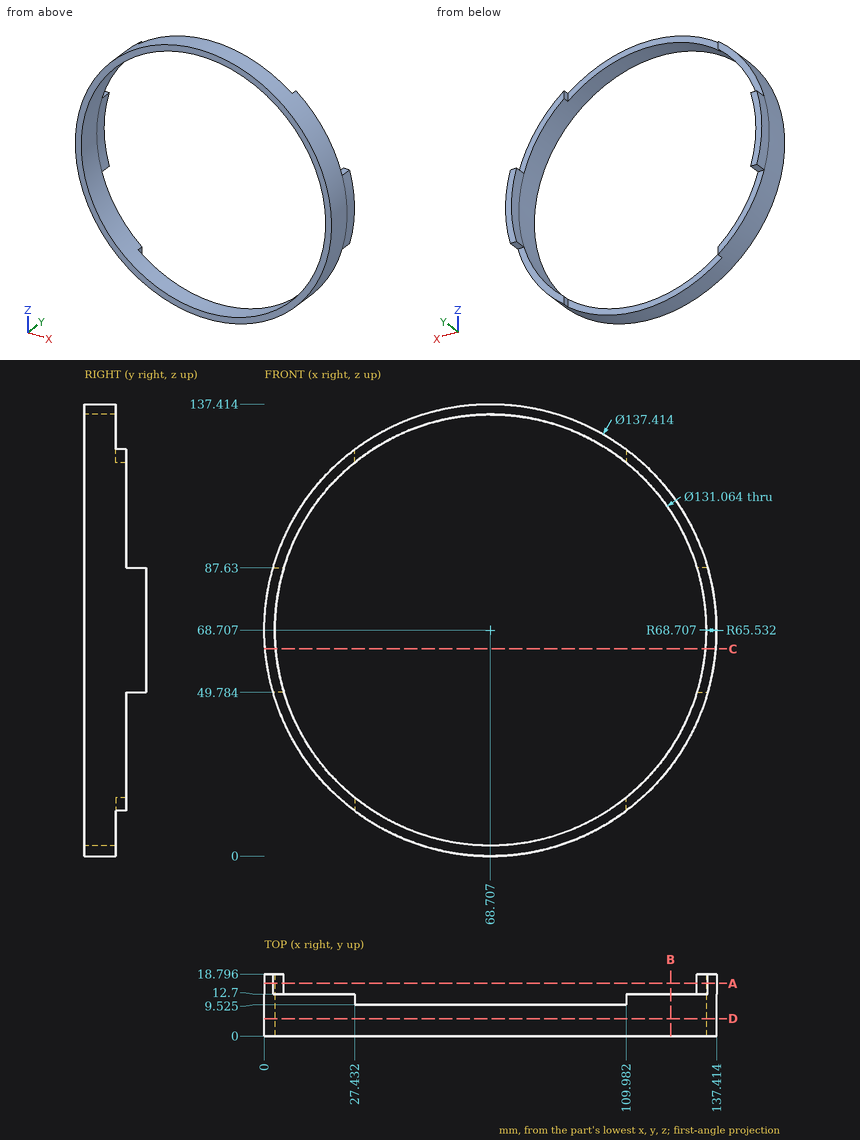
Can you work these out from the drawing? Everything is in mm from the part's minimum corner. Give positions to 0.01 mm unless a question says otherwise; leave off trailing zeros. Order: outer loops, then holes, each group sorted by start corner. A loop starts at its lowest first (then second) coordinate and runs counter-clockwise, first axis right, second up.
Item 1: If we section it at C-C, the plane z = 63: Write out the boundary of the cut face in (x, y), plus the area to 3 significant figures.
Item 2: If we section it at B-B, the plane x = 123.5: Write out the boundary of the cut face in (y, z), plus the area to 3 significant figures.
Item 3: I need wall thicknesses on line 1 (X direction, y = 1.5, z = 89); line 2 (Z direction, x = 14, y = 4.25); line 3 (X direction, y = 2.5, z = 124.5). Which ranges of each line are inside material? Lowest first, please.
Item 4: If we section it at D-D, the plane y = 5.25: Write out the boundary of the cut face in (x, z).
Item 5: I'm going to push flat-ended pins straight in: pin 1 (1.6 mm diameter, centred on y = 11, z = 121.5, fed in from -X); pin 2 (2.5 mm diameter, centred on x = 133, y = 14.5, fed in from -Z); pin 3 (20 mm diameter, centred on x = 17, z = 113, fed in from +Y). Where does each tip first touch, or does it pass through?
Item 6: If we section it at A-A, the plane y = 16: Write out the boundary of the cut face in (x, z), plus the area to 3 significant figures.
Values:
1. outline: (0.24, 0) - (3.42, 0) - (3.42, 18.8) - (0.24, 18.8) - close; (133.99, 0) - (137.18, 0) - (137.18, 18.8) - (133.99, 18.8) - close
1. area: 120 mm2
2. outline: (0, 27.25) - (12.7, 27.25) - (12.7, 32.76) - (0, 32.76) - close; (0, 104.65) - (12.7, 104.65) - (12.7, 110.16) - (0, 110.16) - close
2. area: 140 mm2
3. line 1: x = 3.07 to 6.4, 131.02 to 134.35
3. line 2: z = 27.14 to 32.63, 104.78 to 110.27
3. line 3: x = 28.61 to 34.33, 103.08 to 108.8
4. outline: circle Ø137.41 at (68.71, 68.71); hole circle Ø131.06 at (68.71, 68.71)
5. pin 1: stops at x = 23.79
5. pin 2: stops at z = 49.78
5. pin 3: stops at y = 12.7
6. outline: (2.66, 49.78) - (5.97, 49.78) arc R65.53 cw to (5.97, 87.63) - (2.66, 87.63) arc R68.71 ccw to start; (131.45, 49.78) - (134.76, 49.78) arc R68.71 ccw to (134.76, 87.63) - (131.45, 87.63) arc R65.53 cw to start
6. area: 244 mm2
